from build123d import *

# Parameters (mm, degrees)
SKETCH1_W             = 152.4
SKETCH1_H             = 30.48
BOSS_EXTRUDE1_DEPTH   = 6.35
CUT_EXTRUDE1_DEPTH    = 156.547783334
CUT_EXTRUDE2_DEPTH    = 1.5875
CUT_EXTRUDE3_DEPTH    = 156.547783334
BOSS_EXTRUDE2_DEPTH   = 3.175
F_8_CLEARANCE_HOLE1_D = 4.9149


with BuildPart() as part:
    # Sketch1 → Boss-Extrude1 (new body)
    with BuildSketch(Plane(origin=(0, 0, 0), x_dir=(1, 0, 0), z_dir=(0, 1, 0))):
        with Locations((76.2, 15.24)):
            Rectangle(SKETCH1_W, SKETCH1_H)
    extrude(amount=BOSS_EXTRUDE1_DEPTH)

    # Sketch2 → Cut-Extrude1 (cut, through all)
    with BuildSketch(Plane(origin=(0, 6.35, 0), x_dir=(1, 0, 0), z_dir=(0, 1, 0))):
        with BuildLine():
            Line((12.7, 18.415), (139.7, 18.415))
            ThreePointArc((139.7, 18.415), (142.875, 15.24), (139.7, 12.065))
            Line((139.7, 12.065), (12.7, 12.065))
            ThreePointArc((12.7, 12.065), (9.525, 15.24), (12.7, 18.415))
        make_face()
    extrude(amount=-CUT_EXTRUDE1_DEPTH, mode=Mode.SUBTRACT)

    # Sketch3 → Cut-Extrude2 (cut)
    with BuildSketch(Plane(origin=(0, 6.35, 0), x_dir=(1, 0, 0), z_dir=(0, 1, 0))):
        with BuildLine():
            Line((12.7, 22.493732), (139.7, 22.493732))
            ThreePointArc((139.7, 22.493732), (146.953732, 15.24), (139.7, 7.986268))
            Line((139.7, 7.986268), (12.7, 7.986268))
            ThreePointArc((12.7, 7.986268), (5.446268, 15.24), (12.7, 22.493732))
        make_face()
    extrude(amount=-CUT_EXTRUDE2_DEPTH, mode=Mode.SUBTRACT)

    # Sketch4 → Cut-Extrude3 (cut, through all)
    with BuildSketch(Plane.ZY):
        Polygon((-8.89, 3.175), (-5.715, 0), (0, 0), (0, 3.175), align=None)
    cut_extrude3 = extrude(amount=-CUT_EXTRUDE3_DEPTH, mode=Mode.SUBTRACT)

    # Mirror1: Cut-Extrude3 across plane
    add(cut_extrude3.mirror(Plane(origin=(0, 0, -15.24), x_dir=(1, 0, 0), z_dir=(0, 0, -1))), mode=Mode.SUBTRACT)

    # Sketch8 → Boss-Extrude2 (add)
    with BuildSketch(Plane(origin=(0, 6.35, 0), x_dir=(1, 0, 0), z_dir=(0, 1, 0))):
        with BuildLine():
            Line((0, 0), (-15.24, 0))
            ThreePointArc((-15.24, 0), (-30.48, 15.24), (-15.24, 30.48))
            Line((-15.24, 30.48), (0, 30.48))
            Line((0, 30.48), (0, 0))
        make_face()
    extrude(amount=-BOSS_EXTRUDE2_DEPTH)

    # #8 Clearance Hole1 (through all)
    with Locations(Plane(origin=(0, 6.35, 0), x_dir=(1, 0, 0), z_dir=(0, 1, 0))):
        with Locations((-15.24, 15.24)):
            Hole(F_8_CLEARANCE_HOLE1_D / 2)


solid = part.part
The model under review builds one solid part; all positions refer to its coordinate system, in mm. A direction names the side the tool comes from. Coordinates: 2 decimals unless noted, no trailing zeros. Loops run counter-clockwise (first coordinate to the right, second up) from the corner with the lowest first, then second, coordinate; pieces in that order, holes last. Notation, with made-up numbers: M 43,19.5 L 101,19.5 A15 cw 101,25.5 Z; hole C -39,45 d10. An arc over 180 degrees is marked long. Put each result on its own line as item: value. Start each with the question number.
Q1. Wall thickness on line 1 (X direction, y = 5.7, z = -15.24); line 2 (X direction, y = 4, z = -15.24) (3 decimals); line 3 (Z direction, x = -15.24, y = 4.85): over which ranges is each line inside the solid? List them lowest first.
Q2. Add section D-D (x = -5.5). Write out the cut boundary in (y, z) (3 decimals).
Q3. Add section C-C (y = 2). Write out the cut boundary in (x, z) (3 decimals), and give its area (3 significant figures).
Q4. Add section B-B (z = -15.24). Count the separate pieces of the cut face and the enclosed holes in it, and give its area (3 significant figures).
Q5. Clearance check with flat-ended pins moving along their axes: pin 1 (10 mm diameter, centred on x = 48.5, z = -15.5, fed in from +Y); pin 2 (3.5 mm diameter, centred on y = 1, z = -14.5, fed in from -X); pin 3 (1.4 mm diameter, centred on x = 83.5, y = 2, fed in from -Z) (3 decimals). State where each tip first meets the part, or that it passes through.
Q6. The part is to be moulded in two halves that separate along Z. For faces 6 (the cylindrical face through (-30.476, 4.785, -14.905)), 7 (the flat face through (152.4, 4, -15)), 8 (the cylindrical face through (5.45, 5.57, -15.08)), 9 (the cylindrical face through (-13.29, 4.74, -13.745)), say which applies: +Z half, -Z half, draft (parallel to the pull), parting line (faces both ways), or undercut.
Q7. For faces 1 (the flat face through (70, 5, 0)), 2 (the flat face through (67, 5, -30.48)), 3 (the cylindrical face through (146.95, 5.57, -15.4)), 4 (the cylindrical face through (142.874, 2.415, -15.31)), 5 (the flat face through (0, 2, -15)), list the 3-axis set-ups (+Z, -Z, +X, -X, +Y, -Y) from which the entire face can be reached by the end or side of a thin tool; tool diameter is ignored.
Answers:
1. line 1: x = -30.48 to -17.7, -12.78 to 5.45, 146.95 to 152.4
1. line 2: x = -30.48 to -17.697, -12.783 to 9.525, 142.875 to 152.4
1. line 3: z = -30.48 to -17.7, -12.78 to 0
2. outline: M 3.175,-30.48 L 6.35,-30.48 L 6.35,0 L 3.175,0 Z
3. outline: M 0,-22.765 L 152.4,-22.765 L 152.4,-7.715 L 0,-7.715 Z; hole M 12.7,-18.415 L 139.7,-18.415 A3.175 ccw 139.7,-12.065 L 12.7,-12.065 A3.175 ccw Z
3. area: 1,460 mm^2
4. separate pieces: 3
4. enclosed holes: 0
4. area: 189 mm^2
5. pin 1: stops at y = 4.76
5. pin 2: stops at x = 0
5. pin 3: stops at z = -23.465
6. face 6: parting line
6. face 7: draft
6. face 8: undercut
6. face 9: undercut
7. face 1: +Z, +X, -X, +Y, -Y
7. face 2: -Z, +X, -X, +Y, -Y
7. face 3: +Y
7. face 4: +Y, -Y
7. face 5: +Z, -Z, -X, -Y
